For this review, take the finished solid that the model builds, in its own axes (mm). A direction names the side the tool comes from. Coordinates: 2 decimals unless noted, no trailing zeros. Loops run counter-clockwise (first coordinate to the right, second up) from the corner with the lowest first, then second, coordinate; pieces in that order, holes last. Notation, with made-up numbers: M 82.5,59 L 127.5,59 A7 cw 127.5,68 Z; hole C 14.5,-11 d10. An arc over 180 degrees is marked long. Write item = value, one per line.
from build123d import *

# Parameters (mm, degrees)
F0_W     = 170
F0_H     = 120
F0_W_2   = 166.4
F0_H_2   = 116.4
F1_DEPTH = 165
F3_R     = 54.678141
F4_DEPTH = 159
F6_DEPTH = 4


with BuildPart() as f1:
    # F0 (on Front) → F1 (new body)
    with BuildSketch(Plane.XZ):
        Rectangle(F0_W, F0_H)
        Rectangle(F0_W_2, F0_H_2, mode=Mode.SUBTRACT)
    extrude(amount=F1_DEPTH)


with BuildPart() as f4:
    # F3 (on face) → F4 (new body, symmetric)
    with BuildSketch(Plane.XY.offset(60)):
        with Locations((0, -84.26436)):
            Circle(F3_R)
    extrude(amount=F4_DEPTH, both=True)


with BuildPart() as f1_1:
    add(f1.part)

    # F5: cut F4
    add(f4.part, mode=Mode.SUBTRACT)

    # F0 (on Front) → F6 (join, symmetric)
    with BuildSketch(Plane.XZ):
        Rectangle(F0_W_2, F0_H_2)
    extrude(amount=F6_DEPTH, both=True)


solid = f1_1.part
Q1. For line 1 along X through (y, z) = (-71.5, 17); line 2 along Z through (x, y) = (71.5, -25.5); line 3 along Y through (x, z) = (0, -59.3), list the stretches that pass through material, from the lowest coordinate up.
Solved:
line_1 = -85 to -83.2, 83.2 to 85
line_2 = -60 to -58.2, 58.2 to 60
line_3 = -165 to -138.94, -29.59 to 0
Q2. Draft analysis for pull direction X (two halves, no side actions). For faces 3 (the face through (-39, -45, 60)), 4 (the face through (-11.853, -137.642, -59.087)), 5 (the face through (-85, -81, -1)), state which applies: +X half, -X half, draft (parallel to the pull), parting line (faces both ways), or undercut.
Solved:
face_3 = draft
face_4 = undercut
face_5 = -X half
Q3. Add section B-B (y = -46). Write out the cut boundary in (x, z), and give its area (3 significant figures).
Solved:
outline = M -85,-60 L -39.06,-60 L -39.06,-58.2 L -83.2,-58.2 L -83.2,58.2 L -39.06,58.2 L -39.06,60 L -85,60 Z; M 39.06,-60 L 85,-60 L 85,60 L 39.06,60 L 39.06,58.2 L 83.2,58.2 L 83.2,-58.2 L 39.06,-58.2 Z
area = 750 mm²
Q4. Add section D-D (z = 34.5). Write out the cut boundary in (x, y), and give its area (3 significant figures).
Solved:
outline = M -85,-165 L -83.2,-165 L -83.2,-4 L 83.2,-4 L 83.2,-165 L 85,-165 L 85,0 L 83.2,0 L 83.2,4 L -83.2,4 L -83.2,0 L -85,0 Z
area = 1,930 mm²
Q5. Add section A-A (x = 0). Write out the cut boundary in (y, z).
Solved:
outline = M -165,-60 L -138.94,-60 L -138.94,-58.2 L -165,-58.2 Z; M -165,58.2 L -138.94,58.2 L -138.94,60 L -165,60 Z; M -29.59,-60 L 0,-60 L 0,-58.2 L 4,-58.2 L 4,58.2 L 0,58.2 L 0,60 L -29.59,60 L -29.59,58.2 L -4,58.2 L -4,-58.2 L -29.59,-58.2 Z
Q6. Add section C-C (y = -19). Write out the cut boundary in (x, z).
Solved:
outline = M -85,-60 L 85,-60 L 85,60 L -85,60 Z; hole M -83.2,-58.2 L 83.2,-58.2 L 83.2,58.2 L -83.2,58.2 Z
Q7. Machinability: for faces 1 (the face through (-57, -83, 58.2)), 2 (the face through (85, -81, -1)), which of the approach directions +Z, -Z, +X, -X, +Y, -Y give a long, thin tool a straight path to every point of the face, cutting with its end or side? Answer none if there is none.
Solved:
face_1 = -Y
face_2 = +Z, -Z, +X, +Y, -Y
Q8. For pin 1 Ø5 at (x, z) = (23, -21.5) entering from -Y; pin 2 Ø2 at (y, z) = (1.5, -8) entering from +X, all flat-tipped, find the tip position at first contact; note any pin that passes through.
Solved:
pin_1 = -4
pin_2 = 83.2
